from build123d import *

# Parameters (mm, degrees)
FILLET1_R    = 2.5
SKETCH3_W    = 2.16
SKETCH3_H    = 9.8
SKETCH4_W    = 2.16
SKETCH4_H    = 4.176000402
RECPAT_COUNT = 2
RECPAT_ANGLE = 90


with BuildPart() as part:
    # BodySke → Base-Revolve (revolve)
    with BuildSketch(Plane.XY):
        Polygon((0, 0), (0, 9.15), (0.992391585, 9.15), (5, 5), (50, 5), (50, 0), align=None)
    revolve(axis=Axis((-6.35, 0, 0), (1, 0, 0)))

    # Fillet1
    fillet1_edges = [part.edges().sort_by_distance(p)[0] for p in [
        (5, -5, 0),
    ]]
    fillet(fillet1_edges, radius=FILLET1_R)

    # Sketch3 → Recess section 0
    with BuildSketch(Plane.ZY):
        Rectangle(SKETCH3_W, SKETCH3_H)
    # Sketch4 → Recess section 1
    with BuildSketch(Plane.ZY.offset(-5.64)):
        Rectangle(SKETCH4_W, SKETCH4_H)
    recess = loft(mode=Mode.SUBTRACT)

    # RecPat: Recess ×2 about axis
    recpat_axis = Axis((0, 0, 0), (1, 0, 0))
    for i in range(1, RECPAT_COUNT):
        add(recess.rotate(recpat_axis, i * RECPAT_ANGLE / (RECPAT_COUNT - 1)), mode=Mode.SUBTRACT)

    # RecCorSke → RecessCore (revolve, cut)
    with BuildSketch(Plane.XY):
        Polygon((0, 0), (0, 2.324887219), (5.64, 1.9305), (6.267257474, 0), align=None)
    revolve(axis=Axis((-3.175, 0, 0), (1, 0, 0)), mode=Mode.SUBTRACT)


solid = part.part
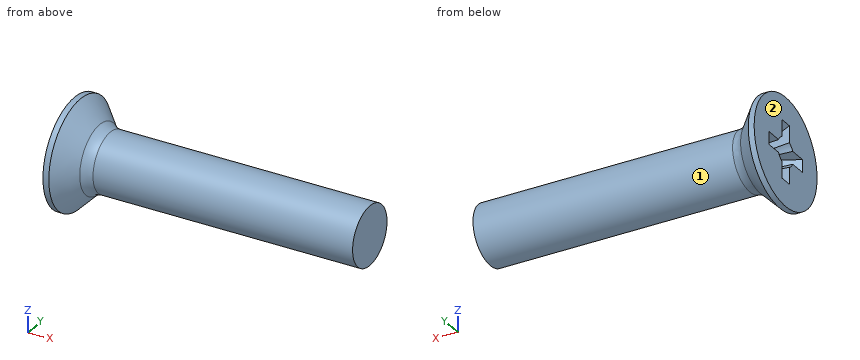
Geometry: final body of the model. Coordinates: model frame, mm. Face numbers are marked on the shaded views. A direction names the side the tool comes from. Give positions to 0.01 mm unless a question says otherwise; leave off trailing zeros. Write each loop counter-clockwise with the first axis right and the second up, starting at its lowest first coordinate (ties: lowest second). Pieces come first, ordered by that corner, then holes.
(1) Ray query, line 1 (Y direction, x = 47.5, z = -0.25); line 2 (Z direction, x = 4, y = -2.5); line 3 (Y direction, x = 14, z = -3.5). Return the intervals inside material, ascending.
(2) Cut plane A-A, the plane x = 33. Return loops of the section in (y, z).
(3) First-contact query: P1, Ø4, axis at x = 35.5, z = 2.5, coming from the -Y side; P2, Ø3, axis at x = 21, y = -3, coming from the -Z side; P3, Ø6, axis at x = 18, z = -4, coming from the -Y side. Flat tips, straight axial feed; report the tip coordinate or a pass-through.
(4) Access query for the marked faces 1 and 2. Directions: +Z, -Z, +X, -X, +Y, -Y. A direction counts if a zero-diameter tool reaches every point of the face in a straight line with its end or side. Return the directions, or none.
Values follow:
1. line 1: y = -4.99 to 4.99
1. line 2: z = -5.49 to -1.08, 1.08 to 5.49
1. line 3: y = -3.57 to 3.57
2. outline: circle Ø10 at (0, 0)
3. P1: stops at y = -4.97
3. P2: stops at z = -4.77
3. P3: stops at y = -4.9
4. face 1: +X
4. face 2: +Z, -Z, -X, +Y, -Y
